from build123d import *

# Parameters (mm, degrees)
F0_R     = 3.175
F1_DEPTH = 6.35


with BuildPart() as f1:
    # F0 (on Top) → F1 (new body)
    with BuildSketch(Plane.XY):
        with BuildLine():
            add(Edge.make_bspline(
                [(12.6999774132, 76.1760478683), (12.6272396661, 37.6088022986), (9.5681586268, 28.3894937776), (25.5841249437, 9.525), (71.131721139, 9.525)],
                knots=[0, 0, 0, 0, 0.4770256041, 1, 1, 1, 1], degree=3))
            ThreePointArc((12.6999774132, 76.1760478683), (0, 88.9), (-12.6999774132, 76.1760478683))
            add(Edge.make_bspline(
                [(-12.6999774132, 76.1760478683), (-12.6272396661, 37.6088022986), (-9.5681586268, 28.3894937776), (-25.5841249437, 9.525), (-71.131721139, 9.525)],
                knots=[0, 0, 0, 0, 0.4770256041, 1, 1, 1, 1], degree=3))
            Line((-71.131721139, 9.525), (-71.131721139, -9.525))
            add(Edge.make_bspline(
                [(-12.6999774132, -76.1760478683), (-12.6272396661, -37.6088022986), (-9.5681586268, -28.3894937776), (-25.5841249437, -9.525), (-71.131721139, -9.525)],
                knots=[0, 0, 0, 0, 0.4770256041, 1, 1, 1, 1], degree=3))
            ThreePointArc((-12.6999774132, -76.1760478683), (0, -88.9), (12.6999774132, -76.1760478683))
            add(Edge.make_bspline(
                [(12.6999774132, -76.1760478683), (12.6272396661, -37.6088022986), (9.5681586268, -28.3894937776), (25.5841249437, -9.525), (71.131721139, -9.525)],
                knots=[0, 0, 0, 0, 0.4770256041, 1, 1, 1, 1], degree=3))
            ThreePointArc((71.131721139, -9.525), (80.656721139, 0), (71.131721139, 9.525))
        make_face()
        with BuildLine():
            ThreePointArc((-6.35, 76.2), (0, 82.55), (6.35, 76.2))
            Line((6.35, 76.2), (6.35, -76.2))
            ThreePointArc((6.35, -76.2), (0, -82.55), (-6.35, -76.2))
            Line((-6.35, -76.2), (-6.35, 76.2))
        make_face(mode=Mode.SUBTRACT)
        with Locations((71.131721139, 0)):
            Circle(F0_R, mode=Mode.SUBTRACT)
    extrude(amount=F1_DEPTH)


solid = f1.part
CAD build for the part. Positions are in the model's coordinates, mm. A direction names the side the tool comes from. Round coordinates to 2 decimals unless told otherwise and drop trailing zeros. Write each loop counter-clockwise with the first axis right and the second up, starting at its lowest first coordinate (ties: lowest second). Pieces come first, ordered by that corner, then holes.
(1) Mould opens along X. For faces 1 (the face through (-71.132, 0, 3)), 2 (the face through (0.14, -82.55, 3.13)), 3 (the face through (11, -6, 0)) say: pulls with the +X half, pulls with the -X half, needs draft (parallel to the pull), parting line crosses it, or undercut.
(2) Probe line 1 along X through (y, z) = (-61, 1.25); line 2 along X through (y, z) = (54, 3); line 3 along Y through (x, z) = (-2, 5.75). List the from-to ranges inside material, lowest first.
(3) Slice it at A-A, the plane x = 0. Write the cut outline in (y, z).
(4) Drop flat-ended pins along their axis: P1, Ø1.9, axis at y = 23, z = 3, coming from the -X side; P2, Ø1, axis at y = 46, z = 4, coming from the -X side; P3, Ø10, axis at x = 71.13, y = 0, coming from the -Z side. Give the stop position or say it passes through.
(5) 3-axis set-ups, long thin cutter, end or side, ignore diameter. For faces 4 (the face through (-0.14, 82.55, 3.13)), 5 (the face through (80.654, -0.209, 3.131)): which of +Z, -Z, +X, -X, +Y, -Y reach the whole face in a straight line?
(6) Slice it at B-B, the plane y = 0. Write the cut outline in (x, z).
(7) Slice it at C-C, the plane z = 5. Count the separate pieces of the cut face and the enclosed holes in it, and give its area (3 significant figures).
From the geometry:
1. face 1: pulls with the -X half
1. face 2: undercut
1. face 3: needs draft
2. line 1: x = -12.59 to -6.35, 6.35 to 12.59
2. line 2: x = -12.49 to -6.35, 6.35 to 12.49
2. line 3: y = -88.74 to -82.23, 82.23 to 88.74
3. outline: (-88.9, 0) - (-82.55, 0) - (-82.55, 6.35) - (-88.9, 6.35) - close; (82.55, 0) - (88.9, 0) - (88.9, 6.35) - (82.55, 6.35) - close
4. P1: stops at x = -16.84
4. P2: stops at x = -12.36
4. P3: stops at z = 0
5. face 4: +Z, -Z
5. face 5: +Z, -Z, +X
6. outline: (-71.13, 0) - (-6.35, 0) - (-6.35, 6.35) - (-71.13, 6.35) - close; (6.35, 0) - (67.96, 0) - (67.96, 6.35) - (6.35, 6.35) - close; (74.31, 0) - (80.66, 0) - (80.66, 6.35) - (74.31, 6.35) - close
7. separate pieces: 1
7. enclosed holes: 2
7. area: 5,500 mm2
